```python
from build123d import *

# Parameters (mm, degrees)
SKETCH_1_W          = 40
SKETCH_1_H          = 40
SKETCH_1_R          = 1.5
EXTRUDE_1_DEPTH     = 20
SKETCH_2_W          = 27.3
SKETCH_2_H          = 17.6
CUT_EXTRUDE_1_DEPTH = 20
SKETCH_3_R          = 13.5
CUT_EXTRUDE_2_DEPTH = 18
SKETCH_4_OUTSIDE_W  = 54
SKETCH_4_OUTSIDE_H  = 54
CUT_EXTRUDE_3_DEPTH = 8
SKETCH_5_OUTSIDE_W  = 54
SKETCH_5_OUTSIDE_H  = 54
CUT_EXTRUDE_4_DEPTH = 58.827329179
SKETCH_6_R          = 13.5
EXTRUDE_2_DEPTH     = 2


with BuildPart() as part:
    # 草图1 → 凸台-拉伸1 (new body)
    with BuildSketch(Plane(origin=(0, 0, 0), x_dir=(1, 0, 0), z_dir=(0, 1, 0))):
        with Locations((20, 20)):
            Rectangle(SKETCH_1_W, SKETCH_1_H)
        with Locations(Location((2.5, 2.5, 0), (0, 0, 270))):
            Circle(SKETCH_1_R, mode=Mode.SUBTRACT)
        with Locations(Location((37.5, 2.5, 0), (0, 0, 270))):
            Circle(SKETCH_1_R, mode=Mode.SUBTRACT)
        with Locations(Location((37.5, 37.5, 0), (0, 0, 270))):
            Circle(SKETCH_1_R, mode=Mode.SUBTRACT)
    extrude(amount=EXTRUDE_1_DEPTH)

    # 草图2 → 切除-拉伸1 (cut)
    with BuildSketch(Plane.ZY):
        with Locations((-25.15, 10)):
            Rectangle(SKETCH_2_W, SKETCH_2_H)
    extrude(amount=-CUT_EXTRUDE_1_DEPTH, mode=Mode.SUBTRACT)

    # 草图3 → 切除-拉伸2 (cut)
    with BuildSketch(Plane(origin=(0, 20, 0), x_dir=(1, 0, 0), z_dir=(0, 1, 0))):
        with Locations(Location((20, 18.7, 0), (0, 0, 270))):
            Circle(SKETCH_3_R)
    extrude(amount=-CUT_EXTRUDE_2_DEPTH, mode=Mode.SUBTRACT)

    # 草图4 outside → 切除-拉伸3 (cut)
    with BuildSketch(Plane(origin=(0, 20, 0), x_dir=(1, 0, 0), z_dir=(0, 1, 0))):
        with Locations((20, 20)):
            Rectangle(SKETCH_4_OUTSIDE_W, SKETCH_4_OUTSIDE_H)
        with BuildLine():
            Line((20, 40), (0, 40))
            Line((0, 40), (0, 20))
            Line((0, 20), (0, 10))
            Line((0, 10), (6.692582543, 5.069740772))
            ThreePointArc((6.692582543, 5.069740772), (38.689638634, 12.879788787), (20, 40))
        make_face(mode=Mode.SUBTRACT)
    extrude(amount=-CUT_EXTRUDE_3_DEPTH, mode=Mode.SUBTRACT)

    # 草图5 outside → 切除-拉伸4 (cut, through all)
    with BuildSketch(Plane(origin=(0, 12, 0), x_dir=(1, 0, 0), z_dir=(0, 1, 0))):
        with Locations((20, 20)):
            Rectangle(SKETCH_5_OUTSIDE_W, SKETCH_5_OUTSIDE_H)
        with BuildLine():
            Line((0, 40), (0, 10))
            add(Edge.make_bspline(
                [(0, 10), (3.638806933, 6.878431862), (0.339826236, 3.758431289)],
                knots=[0, 0, 0, 1, 1, 1], degree=2))
            ThreePointArc((0.339826236, 3.758431289), (1.052952689, 0.461359748), (4.40068463, 0.875993246))
            add(Edge.make_bspline(
                [(11.200276687, 2.039908975), (7.143896711, 3.952452975), (4.40068463, 0.875993246)],
                knots=[0, 0, 0, 1, 1, 1], degree=2))
            ThreePointArc((11.200276687, 2.039908975), (21.144719324, 0.032786432), (30.794624305, 3.163251914))
            add(Edge.make_bspline(
                [(30.794624305, 3.163251914), (34.063948175, 4.035889324), (35.59931537, 0.875993246)],
                knots=[0, 0, 0, 1, 1, 1], degree=2))
            ThreePointArc((35.59931537, 0.875993246), (39.241156707, 0.706017469), (39.180073086, 4.351311542))
            add(Edge.make_bspline(
                [(37.5, 10.317541634), (36.319762019, 6.765651399), (39.180073086, 4.351311542)],
                knots=[0, 0, 0, 1, 1, 1], degree=2))
            ThreePointArc((37.5, 10.317541634), (40, 20), (37.5, 29.682458366))
            add(Edge.make_bspline(
                [(37.5, 29.682458366), (35.925102207, 33.39107959), (39.07643597, 35.559677957)],
                knots=[0, 0, 0, 1, 1, 1], degree=2))
            ThreePointArc((39.07643597, 35.559677957), (39.289523468, 39.245739315), (35.59931537, 39.124006754))
            add(Edge.make_bspline(
                [(29.682458366, 37.5), (33.334347744, 36.215512873), (35.59931537, 39.124006754)],
                knots=[0, 0, 0, 1, 1, 1], degree=2))
            ThreePointArc((29.682458366, 37.5), (25, 39.364916731), (20, 40))
            Line((20, 40), (0, 40))
        make_face(mode=Mode.SUBTRACT)
    extrude(amount=-CUT_EXTRUDE_4_DEPTH, mode=Mode.SUBTRACT)

    # 草图6 → 凸台-拉伸2 (add)
    with BuildSketch(Plane(origin=(0, 2, 0), x_dir=(1, 0, 0), z_dir=(0, 1, 0))):
        with Locations(Location((20, 18.7, 0), (0, 0, 270))):
            Circle(SKETCH_6_R)
    extrude(amount=-EXTRUDE_2_DEPTH)


solid = part.part
```
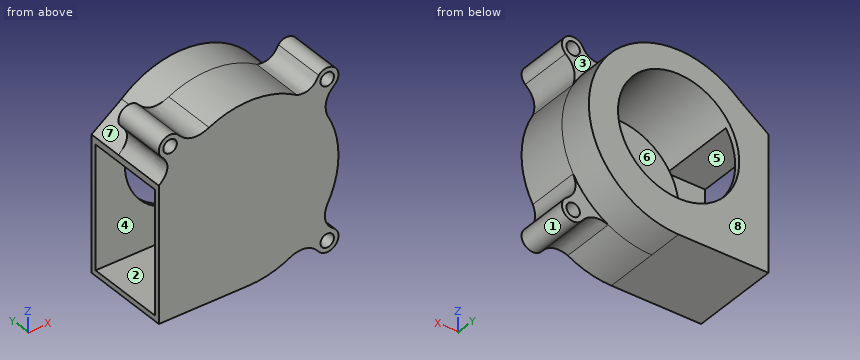
Here's how the part is built. I have some questions about the finished solid (model axes, mm). Face numbers are marked on the shaded views. A direction names the side the tool comes from. Round coordinates to 2 decimals unless told otherwise and drop trailing zeros. Order: outer loops, then holes, each group sorted by start corner. A loop starts at its lowest first (then second) coordinate and runs counter-clockwise, first axis right, second up. Notation, with made-up numbers: (-10.5, 69.25) -> (5.5, 69.25) arc R31 cw to (5.5, 101.25) -> close; hole circle Ø9 at (59.25, 8.25). An arc over 180 degrees is marked (long way). Use a Markdown table: item, result. Add a question column.
(1) Suppose I cut it at A-A, the plane x = 2.5. Please give me the cut outline in (y, z).
(2) For the marked faces 5, 6, 7 and 8, which set-ups out of +Z, -Z, +X, -X, +Y, -Y let a thin tool reach every point of the face, with its end or its side?
(3) I need wall thicknesses on line 1 along Z through (x, y) = (2.5, 8.25); line 2 along Y through (x, z) = (3.5, -17.5); line 3 along Y through (x, z) = (28, -25.5). Which ranges of each line are inside material? Lowest first, please.
(4) Suppose I cut it at B-B, the plane y = 16.5. Please give me the cut outline in (x, z), and give its area (3 significant figures).
(5) Suppose I cut it at C-C, the plane z = -18.7. Please give me the cut outline in (x, y).
(6) If we mould it in two halves opening along Y, with no side actions, what happens to the marked faces 1, 2, 3 and 4? For each: released by +Y, released by -Y, zero draft, split by the parting line, or undercut.
(7) For pin 1 Ø12 at (x, z) = (22.5, -18.5) entering from +Y; pin 2 Ø1 at (y, z) = (12.5, -12.5) entering from +X (3 decimals); pin 3 Ø5 at (x, z) = (37.5, -37.5) entering from +Y, each with a flat end and sliding along its axis, tell me the tip position at first contact or that it passes through.
(8) Suppose I cut it at D-D, the plane x = 18. Please give me the cut outline in (y, z).
Verdict:
| question | item | result |
|---|---|---|
| 1 | outline | (0, -40) -> (20, -40) -> (20, -8.16) -> (12, -8.16) -> (12, -4) -> (0, -4) -> close; (0, -1) -> (12, -1) -> (12, 0) -> (0, 0) -> close; hole (1.2, -38.8) -> (18.8, -38.8) -> (18.8, -11.5) -> (1.2, -11.5) -> close |
| 2 | face 5 | -X |
| 2 | face 6 | +Y |
| 2 | face 7 | +Z, -X, +Y |
| 2 | face 8 | +Z, -Z, +X, -X, +Y |
| 3 | line 1 | -40 to -38.8, -11.5 to -4, -1 to 0 |
| 3 | line 2 | 0 to 1.2, 18.8 to 20 |
| 3 | line 3 | 0 to 2 |
| 4 | outline | (0, -40) -> (20, -40) arc R20 ccw (long way) to (6.69, -5.07) -> (0, -10) -> (0, -11.5) -> (8.58, -11.5) arc R13.5 cw (long way) to (20, -32.2) -> (20, -38.8) -> (0, -38.8) -> close |
| 4 | area | 474 mm2 |
| 5 | outline | (0, 0) -> (39.96, 0) -> (39.96, 20) -> (33.5, 20) -> (33.5, 2) -> (6.5, 2) -> (6.5, 1.2) -> (0, 1.2) -> close; (0, 18.8) -> (6.5, 18.8) -> (6.5, 20) -> (0, 20) -> close |
| 6 | face 1 | zero draft |
| 6 | face 2 | undercut |
| 6 | face 3 | released by +Y |
| 6 | face 4 | undercut |
| 7 | pin 1 | y = 2 |
| 7 | pin 2 | x = 38.735 |
| 7 | pin 3 | y = 12 |
| 8 | outline | (0, -40) -> (20, -40) -> (20, -32.05) -> (18.8, -32.05) -> (18.8, -38.8) -> (1.2, -38.8) -> (1.2, -32.05) -> (2, -32.05) -> (2, -5.35) -> (20, -5.35) -> (20, -0.1) -> (0, -0.1) -> close |
